from build123d import *

# Parameters (mm, degrees)
BOSS_EXTRUDE1_DEPTH        = 28.575
CUT_EXTRUDE1_DEPTH         = 21.59
F_8_0_199_DIAMETER_HOLE1_D = 5.0546
HOLE1_D                    = 50.8
CHAMFER1_SIZE              = 26.940768363


with BuildPart() as part:
    # Sketch1 → Boss-Extrude1 (new body)
    with BuildSketch(Plane(origin=(0, 28.575, 0), x_dir=(1, 0, 0), z_dir=(0, 1, 0))):
        Polygon((127, 273.05), (-19.05, 127), (127, -19.05), (273.05, 127), align=None)
    extrude(amount=-BOSS_EXTRUDE1_DEPTH)

    # Sketch2 → Cut-Extrude1 (cut)
    with BuildSketch(Plane(origin=(0, 28.575, 0), x_dir=(-1, 0, 0), z_dir=(0, 1, 0))):
        with BuildLine():
            ThreePointArc((-149.467157898, -88.646), (-158.430896424, -95.569103576), (-165.354, -104.532842102))
            ThreePointArc((-165.354, -104.532842102), (-248.158, -127), (-165.354, -149.467157898))
            ThreePointArc((-165.354, -149.467157898), (-158.430896424, -158.430896424), (-149.467157898, -165.354))
            ThreePointArc((-149.467157898, -165.354), (-127, -248.158), (-104.532842102, -165.354))
            ThreePointArc((-104.532842102, -165.354), (-95.569103576, -158.430896424), (-88.646, -149.467157898))
            ThreePointArc((-88.646, -149.467157898), (-5.842, -127), (-88.646, -104.532842102))
            ThreePointArc((-88.646, -104.532842102), (-95.569103576, -95.569103576), (-104.532842102, -88.646))
            ThreePointArc((-104.532842102, -88.646), (-127, -5.842), (-149.467157898, -88.646))
        make_face()
    extrude(amount=-CUT_EXTRUDE1_DEPTH, mode=Mode.SUBTRACT)

    # #8 (0.199) Diameter Hole1 (through all)
    with Locations(Plane(origin=(0, 28.575, 0), x_dir=(1, 0, 0), z_dir=(0, 1, 0))):
        with Locations((180.881536726, 183.247438789), (180.881536726, 70.752561211), (70.752561211, 73.118463274), (70.752561211, 180.881536726)):
            Hole(F_8_0_199_DIAMETER_HOLE1_D / 2)

    # Hole1 (through all)
    with Locations(Plane(origin=(0, 6.985, 0), x_dir=(1, 0, 0), z_dir=(0, 1, 0))):
        with Locations((127, 127), (127, 203.708), (50.292, 127), (127, 50.292), (203.708, 127)):
            Hole(HOLE1_D / 2)

    # Chamfer1
    chamfer1_edges = [part.edges().sort_by_distance(p)[0] for p in [
        (273.05, 14.2875, -127),
        (127, 14.2875, 19.05),
        (-19.05, 14.2875, -127),
        (127, 14.2875, -273.05),
    ]]
    chamfer(chamfer1_edges, length=CHAMFER1_SIZE)


solid = part.part
Input: part model. Units: mm. Frame: model coordinates. A direction names the side the tool comes from. Give positions to 0.01 mm unless a question says otherwise; leave off trailing zeros. Write each loop counter-clockwise with the first axis right and the second up, starting at its lowest first coordinate (ties: lowest second). Pieces come first, ordered by that corner, then holes.
Q1. Pull-direction query (Z, two-part tool) for faces 1 (the face through (103.54, 3.44, -40.56)), 2 (the face through (0, 14, -127)), 3 (the face through (200.78, 14.49, -199.27)); classes: pulls with the +Z half, pulls with the -Z half, needs draft (parallel to the pull), parting line crosses it, or undercut.
Q2. First-contact query: P1, Ø3, axis at x = 180.88, z = -183.25, coming from the -Y side; P2, Ø2, axis at x = 65.5, y = 23.5, coming from the -Z side; P3, Ø12, axis at x = 181.5, y = 16, coming from the +Z side; P4, Ø2, axis at y = 17, z = -52, coming from the +X side. Flat tips, straight axial feed; report the tip coordinate or a pass-through.
Q3. Material intervals for probe 1 along X at (y, z) = (1.5, -127); probe 2 along Z at (x, y) = (127, 4.75); probe 3 along X at (y, z) = (16, -127), sorted ascending.
Q4. Section B-B, the plane z = -127. Output: boundary loops of the cut face in (x, y) (3 decimals), plus the area to 3 significant figures.
Q5. Section D-D, the plane y = 21.75. Output: boundary loops of the cut face in (x, z), plus the area to 3 significant figures.
Q6. Set-up query: faces 4 (the face through (128.62, 17.93, -248.13)), 5 (the face through (102.773, 3.444, -134.629)). Return all of +Z, -Z, +X, -X, +Y, -Y with unobstructed straight access to the full face (end or side cutting, diameter ignored); none if empty.
Q7. Section A-A, the plane x = 127. Output: boundary loops of the cut face in (y, z) (3 decimals), plus the area to 3 significant figures.
Q8. Section C-C, the plane x = 214.5. Output: boundary loops of the cut face in (y, z) (3 decimals).
Filled in:
1. face 1: undercut
1. face 2: needs draft
1. face 3: pulls with the -Z half
2. P1: passes through
2. P2: stops at z = -212.55
2. P3: stops at z = -29.45
2. P4: stops at x = 199.05
3. probe 1: x = 0 to 24.89, 75.69 to 101.6, 152.4 to 178.31, 229.11 to 254
3. probe 2: z = -254 to -229.11, -178.31 to -152.4, -101.6 to -75.69, -24.89 to 0
3. probe 3: x = 0 to 5.84, 248.16 to 254
4. outline: (0, 0) - (24.892, 0) - (24.892, 6.985) - (5.842, 6.985) - (5.842, 28.575) - (0, 28.575) - close; (75.692, 0) - (101.6, 0) - (101.6, 6.985) - (75.692, 6.985) - close; (152.4, 0) - (178.308, 0) - (178.308, 6.985) - (152.4, 6.985) - close; (229.108, 0) - (254, 0) - (254, 28.575) - (248.158, 28.575) - (248.158, 6.985) - (229.108, 6.985) - close
4. area: 962 mm2
5. outline: (0, -146.05) - (107.95, -254) - (146.05, -254) - (254, -146.05) - (254, -107.95) - (146.05, 0) - (107.95, 0) - (0, -107.95) - close; hole circle Ø5.05 at (70.75, -180.88); hole circle Ø5.05 at (70.75, -73.12); hole (88.65, -149.47) arc R44.45 ccw to (104.53, -165.35) arc R44.45 ccw (long way) to (149.47, -165.35) arc R44.45 ccw to (165.35, -149.47) arc R44.45 ccw (long way) to (165.35, -104.53) arc R44.45 ccw to (149.47, -88.65) arc R44.45 ccw (long way) to (104.53, -88.65) arc R44.45 ccw to (88.65, -104.53) arc R44.45 ccw (long way) to start; hole circle Ø5.05 at (180.88, -183.25); hole circle Ø5.05 at (180.88, -70.75)
5. area: 11,600 mm2
6. face 4: +Y
6. face 5: +Y, -Y
7. outline: (0, -254) - (28.575, -254) - (28.575, -248.158) - (6.985, -248.158) - (6.985, -229.108) - (0, -229.108) - close; (0, -178.308) - (6.985, -178.308) - (6.985, -152.4) - (0, -152.4) - close; (0, -101.6) - (6.985, -101.6) - (6.985, -75.692) - (0, -75.692) - close; (0, -24.892) - (6.985, -24.892) - (6.985, -5.842) - (28.575, -5.842) - (28.575, 0) - (0, 0) - close
7. area: 962 mm2
8. outline: (0, -185.55) - (28.575, -185.55) - (28.575, -170.12) - (6.985, -170.12) - (6.985, -149.993) - (0, -149.993) - close; (0, -104.007) - (6.985, -104.007) - (6.985, -83.88) - (28.575, -83.88) - (28.575, -68.45) - (0, -68.45) - close
